Verification items for the finished model (mm, model axes). Coordinates: 2 decimals unless noted, no trailing zeros.
Q1. Go/stop test with flat-tipped pins: P1, Ø1, axis at x = 2, y = 64.5, coming from the +Z side; P2, Ø7.5, axis at x = -9, z = 3.5, coming from the +Y side; P3, Ø4, axis at x = -18.5, y = 76, coming from the -Z side. Record where each tip stops, or that it passes through.
Q2. Material ranges on probe 1 along X at (y, z) = (49.5, -7.5); probe 2 along Z at (x, y) = (-19.5, 31); probe 3 along Y at (x, z) = (7.5, 2), recorded low to high.
Q3. Mould release check, pull along X, two halves, no side actions. Record for faces 1 (the face through (0, 85.065, 18)), 2 (the face through (0, -0.237, 0)), 3 (the face through (0, 0, 0)): +X half, -X half, draft (parallel to the pull), parting line (faces both ways), or undercut.
Autodesk Inventor part; units mm, degrees
ref_plane "Work Plane1" through (0, 84.6667, 0) normal (0, 1, 0) x (-1, 0, 0)
ref_plane "YZ Plane" through (0, 0, 0) normal (1, 0, 0) x (0, 1, 0)
ref_plane "XY Plane" through (0, 0, 0) normal (0, 0, 1) x (1, 0, 0)
sketch "Sketch1" plane through (0, 0, 0) normal (0, 1, 0) x (-1, 0, 0)
  line L0 (17.8888, -12.7) -> (0, -12.7)
  line L1 (0, 12.7) -> (17.8888, 12.7)
  line L2 (19.05, 11.5388) -> (19.05, -11.5388)
  arc A0 (17.8888, -12.7) -> (19.05, -11.5388) centre (17.8888, -11.5388) ccw
  line L3 (0, -12.7) -> (0, 12.7) construction
  arc A1 (19.05, 11.5388) -> (17.8888, 12.7) centre (17.8888, 11.5388) ccw
  line L4 (17.8888, -12.4629) -> (0, -12.4629)
  line L5 (0, 12.4629) -> (17.8888, 12.4629)
  line L6 (18.8129, 11.5388) -> (18.8129, -11.5388)
  arc A2 (17.8888, -12.4629) -> (18.8129, -11.5388) centre (17.8888, -11.5388) ccw
  arc A3 (18.8129, 11.5388) -> (17.8888, 12.4629) centre (17.8888, 11.5388) ccw
  line L7 (-17.8888, -12.7) -> (0, -12.7)
  line L8 (0, 12.7) -> (-17.8888, 12.7)
  line L9 (-19.05, 11.5388) -> (-19.05, -11.5388)
  arc A4 (-19.05, -11.5388) -> (-17.8888, -12.7) centre (-17.8888, -11.5388) ccw
  arc A5 (-17.8888, 12.7) -> (-19.05, 11.5388) centre (-17.8888, 11.5388) ccw
  line L10 (-17.8888, -12.4629) -> (0, -12.4629)
  line L11 (0, 12.4629) -> (-17.8888, 12.4629)
  line L12 (-18.8129, 11.5388) -> (-18.8129, -11.5388)
  arc A6 (-18.8129, -11.5388) -> (-17.8888, -12.4629) centre (-17.8888, -11.5388) ccw
  arc A7 (-17.8888, 12.4629) -> (-18.8129, 11.5388) centre (-17.8888, 11.5388) ccw
  point P0 (0, 0)
  point P1 (0, 0)
  dimension "d2" = 0.2371
  dimension "d3" = 0.2371
  dimension "d4" = 0.2371
  dimension "d6" = 19.05
  dimension "d7" = 25.4
  dimension "d17" = 0.9241
extrude "bottom of bin" add sketch "Sketch1" against normal blind 0.2371 contours L0 L7 A4 L9 A5 L8 L1 A1 L2 A0 | L4 L10 A6 L12 A7 L11 L5 A3 L6 A2
ref_plane "Work Plane1" through (0, 84.6667, 0) normal (0, 1, 0) x (-1, 0, 0)
sketch "Sketch2" plane through (0, 84.6667, 0) normal (0, 1, 0) x (-1, 0, 0)
  line L0 (0, -16.9333) -> (22.3592, -16.9333)
  line L1 (23.2833, -16.0092) -> (23.2833, 16.0092)
  line L2 (22.3592, 16.9333) -> (0, 16.9333)
  line L3 (17.8888, -12.7) -> (-17.8888, -12.7)
  line L4 (17.8888, 12.7) -> (-17.8888, 12.7)
  line L5 (19.05, -11.5388) -> (19.05, 11.5388)
  line L6 (0, -17.1704) -> (22.3592, -17.1704)
  line L7 (23.5204, -16.0092) -> (23.5204, 16.0092)
  line L8 (22.3592, 17.1704) -> (0, 17.1704)
  arc A0 (22.3592, -16.9333) -> (23.2833, -16.0092) centre (22.3592, -16.0092) ccw
  arc A1 (23.2833, 16.0092) -> (22.3592, 16.9333) centre (22.3592, 16.0092) ccw
  arc A2 (23.5204, 16.0092) -> (22.3592, 17.1704) centre (22.3592, 16.0092) ccw
  arc A3 (22.3592, -17.1704) -> (23.5204, -16.0092) centre (22.3592, -16.0092) ccw
  line L9 (0, -8.1161) -> (0, 0) construction
  line L10 (0, -16.9333) -> (-22.3592, -16.9333)
  line L11 (-23.2833, -16.0092) -> (-23.2833, 16.0092)
  line L12 (-22.3592, 16.9333) -> (0, 16.9333)
  line L13 (0, -17.1704) -> (-22.3592, -17.1704)
  line L14 (-23.5204, -16.0092) -> (-23.5204, 16.0092)
  line L15 (-22.3592, 17.1704) -> (0, 17.1704)
  arc A4 (-23.2833, -16.0092) -> (-22.3592, -16.9333) centre (-22.3592, -16.0092) ccw
  arc A5 (-22.3592, 16.9333) -> (-23.2833, 16.0092) centre (-22.3592, 16.0092) ccw
  arc A6 (-22.3592, 17.1704) -> (-23.5204, 16.0092) centre (-22.3592, 16.0092) ccw
  arc A7 (-23.5204, -16.0092) -> (-22.3592, -17.1704) centre (-22.3592, -16.0092) ccw
  point P0 (0, 0)
  dimension "d11" = 4.2333
  dimension "d12" = 4.2333
  dimension "d13" = 4.2333
  dimension "d14" = 0.2371
  dimension "d15" = 0.2371
  dimension "d16" = 0.2371
  dimension "d18" = 0.9241
  dimension "d19" = 0.9241
loft "loft make" add profiles "Sketch2", "Sketch1" contours L10 A4 L11 A5 L12 L2 A1 L1 A0 L0 | L13 A7 L14 A6 L15 L8 A2 L7 A3 L6 / L0 L7 A4 L9 A5 L8 L1 A1 L2 A0 | L4 L10 A6 L12 A7 L11 L5 A3 L6 A2
loft "loft cut" cut profiles "Sketch2", "Sketch1" contours L10 A4 L11 A5 L12 L2 A1 L1 A0 L0 / L4 L10 A6 L12 A7 L11 L5 A3 L6 A2
sketch "Sketch3" plane through (0, 0, 0) normal (1, 0, 0) x (0, 1, 0)
  line L0 (84.6667, 16.9333) -> (0, 12.4629)
  arc A0 (84.6667, 16.9333) -> (85.3017, 17.6027) centre (84.6313, 17.6027) ccw
  line L1 (85.3017, 17.6027) -> (85.3017, 18.415)
  arc A1 (84.6667, 17.1704) -> (85.0651, 17.6027) centre (84.6313, 17.6027) ccw
  arc A2 (85.3017, 18.415) -> (84.6667, 19.05) centre (84.6667, 18.415) ccw
  line L2 (84.6667, 19.05) -> (84.533, 19.05) construction
  line L3 (84.6667, 19.05) -> (84.6667, 18.8134)
  line L4 (85.0651, 17.6027) -> (85.0651, 18.415)
  arc A3 (85.0651, 18.415) -> (84.6667, 18.8134) centre (84.6667, 18.415) ccw
  line L5 (84.6667, 17.1704) -> (84.6667, 16.0092)
  line L6 (84.6667, 16.9333) -> (84.6667, 17.1704)
  point P0 (0, 0)
  dimension "d28" = 2.1167
  dimension "d29" = 0.635
sweep "lip rim" add profiles "Sketch3" path "Sketch2" path curves L8 A2 L7 A3 L6 L13 A7 L14 A6 L15
equation "\"d3\" = d2"
equation "\"d4\" = d2"
equation "\"d8\" = d2"
equation "\"d12\" = d11"
equation "\"d13\" = d11"
equation "\"d14\" = d2"
equation "\"d15\" = d2"
equation "\"d16\" = d2"
equation "\"d18\" = d17"
equation "\"d19\" = d17"
properties part number "recycle and trash bin"
Geometry check:
1. P1: stops at z = 16.13
1. P2: stops at y = 0
1. P3: stops at z = -16.82
2. probe 1: x = -21.66 to -21.43, 21.43 to 21.66
2. probe 2: z = -14.34 to -14.1, 14.1 to 14.34
2. probe 3: y = -0.24 to 0
3. face 1: undercut
3. face 2: draft
3. face 3: undercut
